```python
from build123d import *

# Parameters (mm, degrees)
F2_SIZE  = 3
F3_R     = 7.5
F4_DEPTH = 12.9
F5_R     = 3
F6_R     = 1
F7_DEPTH = 25


with BuildPart() as f1:
    # F0 (on Front) → F1 (revolve)
    with BuildSketch(Plane.XZ):
        Polygon((0, 17), (0, 0), (10.35, 0), (13.35, 0), (13.35, 2), (10.35, 2), (10.35, 4), (9.85, 4), (9.85, 5), (10.35, 5), (10.35, 7), (9.85, 7), (9.85, 8), (10.35, 8), (10.35, 10), (9.85, 10), (9.85, 11), (10.35, 11), (10.35, 17), align=None)
    revolve(axis=Axis((0, 0, 12.16054), (0, 0, 1)))

    # F2
    f2_edges = [f1.edges().sort_by_distance(p)[0] for p in [
        (-10.35, 0, 17),
    ]]
    chamfer(f2_edges, length=F2_SIZE)

    # F3 (on face) → F4 (cut)
    with BuildSketch(Plane.XY.offset(17)):
        Circle(F3_R)
    extrude(amount=-F4_DEPTH, mode=Mode.SUBTRACT)

    # F5
    f5_edges = [f1.edges().sort_by_distance(p)[0] for p in [
        (-7.5, 0, 4.1),
    ]]
    fillet(f5_edges, radius=F5_R)

    # F6 (on face) → F7 (cut)
    with BuildSketch(Plane(origin=(0, 0, 0), x_dir=(1, 0, 0), z_dir=(0, 0, -1))):
        Circle(F6_R)
    extrude(amount=-F7_DEPTH, mode=Mode.SUBTRACT)


solid = f1.part
```
Here's how the part is built. I have some questions about the finished solid (model axes, mm). A direction names the side the tool comes from. Give positions to 0.01 mm unless a question says otherwise; leave off trailing zeros. Order: outer loops, then holes, each group sorted by start corner. A loop starts at its lowest first (then second) coordinate and runs counter-clockwise, first axis right, second up. Notation, with made-up numbers: (24.25, -10.75) - (57.25, -10.75) arc R5 ccw to (57.25, -3.75) - close; hole circle Ø7 at (-28, 31.25). An arc over 180 degrees is marked (long way). Answer as a JSON object with one key per item and string values. Group by question number.
Item 1: Please list where these lines run through material, in increasing order: probe 1 along Y at (x, z) = (0, 2.7); probe 2 along Z at (x, y) = (-9.5, 3.5); probe 3 along Y at (x, z) = (0, 9.75).
Item 2: If we section it at B-B on y = 11: Please give me the cut outline in (x, z).
Item 3: If we section it at A-A on z = 1.5: Please give me the cut outline in (x, y).
Item 4: Which directions (+Z, -Z, +X, -X, +Y, -Y) give clear straight access to the entire face, cutting with the end or side of a thin tool? Please do faces 1 (the cylindrical face through (-8.21, -6.3, 6.01)), 2 (the flat face through (0, -3, 0)), 3 (the flat face through (0, -10, 4)).
Item 5: If we section it at C-C on z = 12.75: Please give me the cut outline in (x, y).
Item 6: For P1, Ø3, axis at x = -5, y = -1, coming from the -Z side; P2, Ø4, axis at x = 7.5, z = 14, coming from the +Y side; P3, Ø5, axis at x = 2, z = 10, coming from the -Y side; P4, Ø3, axis at y = -5.5, z = 5.5, coming from the -X side, each with a flat end and sliding along its axis, tell me the tip position at first contact or that it passes through.
Item 7: If we mould it in two halves opening along X, with no side actions, what happens to faces 4 (the cylindrical face through (-8.21, -6.3, 3.01)), 5 (the flat face through (0, -10, 5)), 6 (the flat face through (1, -1, 4.1)), 7 (the cylindrical face through (-7.493, 0.33, 12.043))? For each: pulls with the +X half, pulls with the -X half, needs draft (parallel to the pull), parting line crosses it, or undercut.
Result set:
{
 "1": {"probe 1": "-10.35 to -1, 1 to 10.35", "probe 2": "0 to 4, 5 to 7, 8 to 10, 11 to 14.23", "probe 3": "-10.35 to -7.5, 7.5 to 10.35"},
 "2": {"outline": "(-7.56, 0) - (7.56, 0) - (7.56, 2) - (-7.56, 2) - close"},
 "3": {"outline": "circle Ø26.7 at (0, 0); hole circle Ø2 at (0, 0)"},
 "4": {"face 1": "+Z", "face 2": "-Z, +X, -X, +Y, -Y", "face 3": "none"},
 "5": {"outline": "circle Ø20.7 at (0, 0); hole circle Ø15 at (0, 0)"},
 "6": {"P1": "z = 0", "P2": "y = 8.77", "P3": "y = -10.35", "P4": "x = -9.55"},
 "7": {"face 4": "parting line crosses it", "face 5": "needs draft", "face 6": "undercut", "face 7": "undercut"}
}
